Read the model definition and answer for the solid it produces. Units are mm, in the model's axes. A direction names the side the tool comes from. Coordinates: 2 decimals unless noted, no trailing zeros. Loops run counter-clockwise (first coordinate to the right, second up) from the corner with the lowest first, then second, coordinate; pieces in that order, holes last. Notation, with made-up numbers: M 6.25,0 L 23.25,0 A18 ccw 23.25,31 Z; hole C -22.5,-7.5 d8. An arc over 180 degrees is marked long. Use one line per item in the form item = value. Start each with the question number.
1. The part is cut by section B-B (x = 122.5). Give the vertices of the cut face in (y, z) (3 decimals), plus the area to 3 significant figures.
2. The part is cut by section D-D (z = -32.5). Give the vertices of the cut face in (x, y).
3. The part is cut by section A-A (y = 35). Give the vertices of the cut face in (x, z) (3 decimals), plus the area to 3 significant figures.
4. Find the intervals of material crossed by probe 1 along Z at (x, y) = (30, 36) (3 decimals); probe 2 along Y at (x, z) = (71.12, 4); probe 3 along Y at (x, z) = (71.12, 1.5), in increasing order. Write a range as [from, to].
5. For a pull along Y with two mould halves and no side action, classify faces 5 (the flat face through (35, 35, -9.525)), 6 (the cylindrical face through (166.765, 28.206, -10.671)), 7 (the flat face through (106, 31.75, -19)) as released by +Y, released by -Y, zero draft, split by the parting line, or undercut.
6. A tool of negligible diameter and unlimited length cuts with its end or side. For faces 1 (the cylindrical face through (63.684, 34.881, -27.429)), 2 (the cylindrical face through (61.597, 22.47, 4.507)), 3 (the flat face through (71.1, 6.6, 2.54)), 4 (the flat face through (84.264, 7, 4)), from which of +Z, -Z, +X, -X, +Y, -Y can it reach the whole face along a straight path? Write none if from no direction.
7. Flat-ended cylindrical pins translate along their axes: pin 1 (8 mm diameter, centred on x = 41, y = 12, fed in from +Z); pin 2 (5 mm diameter, centred on y = 34.5, z = -18.5, fed in from +X); pin 3 (10 mm diameter, centred on y = 6.5, z = 3, fed in from +X); pin 4 (5 mm diameter, centred on x = 20, z = 3.5, fed in from +Y). Find the tip coordinate at first contact, or state that the pin passes through.
from build123d import *

# Parameters (mm, degrees)
BOSS_EXTRUDE1_DEPTH = 38.1
SKETCH2_R           = 10.8585
CUT_EXTRUDE1_DEPTH  = 25.4
SKETCH3_R           = 10.8585
CUT_EXTRUDE2_DEPTH  = 25.4
FILLET1_R           = 10
FILLET2_R           = 10
SKETCH5_W           = 26.289
SKETCH5_H           = 26.289
BOSS_EXTRUDE2_DEPTH = 8.89
SKETCH6_R           = 8.0645
CUT_EXTRUDE3_DEPTH  = 6.35
SKETCH7_R           = 6.35
CUT_EXTRUDE4_DEPTH  = 5.08
FILLET3_R           = 12.7
SKETCH8_W           = 58.1046987
SKETCH8_H           = 19.05
CUT_EXTRUDE5_DEPTH  = 6.35
FILLET4_R           = 3.81


with BuildPart() as part:
    # Sketch1 → Boss-Extrude1 (new body)
    with BuildSketch(Plane(origin=(0, 0, 0), x_dir=(1, 0, 0), z_dir=(0, 1, 0))):
        Polygon((0, 0), (142.24, 0), (158.021536726, -15.781536726), (184.96230509, 11.159231637), (158.021536726, 38.1), (-15.781536726, 38.1), (-42.72230509, 11.159231637), (-15.781536726, -15.781536726), align=None)
    extrude(amount=BOSS_EXTRUDE1_DEPTH)

    # Sketch2 → Cut-Extrude1 (cut)
    with BuildSketch(Plane(origin=(-15.781536726, 0, 15.781536726), x_dir=(0.7071067811865477, 0, 0.7071067811865475), z_dir=(-0.7071067811865475, 0, 0.7071067811865477))):
        with Locations((-19.05, 19.05)):
            Circle(SKETCH2_R)
    extrude(amount=-CUT_EXTRUDE1_DEPTH, mode=Mode.SUBTRACT)

    # Sketch3 → Cut-Extrude2 (cut)
    with BuildSketch(Plane(origin=(86.901536726, 0, 86.901536726), x_dir=(0.7071067811865478, 0, -0.7071067811865474), z_dir=(0.7071067811865474, 0, 0.7071067811865478))):
        with Locations((119.628868556, 19.05)):
            Circle(SKETCH3_R)
    extrude(amount=-CUT_EXTRUDE2_DEPTH, mode=Mode.SUBTRACT)

    # Fillet1
    fillet1_edges = [part.edges().sort_by_distance(p)[0] for p in [
        (142.24, 19.05, 0),
        (0, 19.05, 0),
    ]]
    fillet(fillet1_edges, radius=FILLET1_R)

    # Fillet2
    fillet2_edges = [part.edges().sort_by_distance(p)[0] for p in [
        (-15.781536726, 19.05, -38.1),
        (158.021536726, 19.05, -38.1),
    ]]
    fillet(fillet2_edges, radius=FILLET2_R)

    # Sketch5 → Boss-Extrude2 (add)
    with BuildSketch(Plane.XY):
        with Locations((71.12, 13.1445)):
            Rectangle(SKETCH5_W, SKETCH5_H)
    extrude(amount=BOSS_EXTRUDE2_DEPTH)

    # Sketch6 → Cut-Extrude3 (cut)
    with BuildSketch(Plane.XY.offset(8.89)):
        with Locations((71.12, 13.1445)):
            Circle(SKETCH6_R)
    extrude(amount=-CUT_EXTRUDE3_DEPTH, mode=Mode.SUBTRACT)

    # Sketch7 → Cut-Extrude4 (cut)
    with BuildSketch(Plane.XY.offset(2.54)):
        with Locations((71.12, 13.1445)):
            Circle(SKETCH7_R)
    extrude(amount=-CUT_EXTRUDE4_DEPTH, mode=Mode.SUBTRACT)

    # Fillet3
    fillet3_edges = [part.edges().sort_by_distance(p)[0] for p in [
        (57.9755, 26.289, 4.445),
        (84.2645, 26.289, 4.445),
    ]]
    fillet(fillet3_edges, radius=FILLET3_R)

    # Sketch8 → Cut-Extrude5 (cut)
    with BuildSketch(Plane(origin=(0, 38.1, 0), x_dir=(1, 0, 0), z_dir=(0, 1, 0))):
        with Locations((35.71765065, 19.05)):
            Rectangle(SKETCH8_W, SKETCH8_H)
        with Locations((106.52234935, 19.05)):
            Rectangle(SKETCH8_W, SKETCH8_H)
    extrude(amount=-CUT_EXTRUDE5_DEPTH, mode=Mode.SUBTRACT)

    # Fillet4
    fillet4_edges = [part.edges().sort_by_distance(p)[0] for p in [
        (6.6653013, 34.925, -9.525),
        (6.6653013, 34.925, -28.575),
        (64.77, 34.925, -28.575),
        (64.77, 34.925, -9.525),
        (135.5746987, 34.925, -28.575),
        (135.5746987, 34.925, -9.525),
        (77.47, 34.925, -9.525),
        (77.47, 34.925, -28.575),
    ]]
    fillet(fillet4_edges, radius=FILLET4_R)


solid = part.part
Computed values:
q1.outline = M 0,-38.1 L 38.1,-38.1 L 38.1,-28.575 L 31.75,-28.575 L 31.75,-9.525 L 38.1,-9.525 L 38.1,0 L 0,0 Z
q1.area = 1,330 mm²
q2.outline = M -21.38,0 L 163.62,0 L 163.62,38.1 L -21.38,38.1 Z
q3.outline = M -42.722,-11.159 L -18.71,-35.171 A10 ccw -11.639,-38.1 L 153.879,-38.1 A10 ccw 160.95,-35.171 L 184.962,-11.159 L 158.022,15.782 L 145.169,2.929 A10 cw 138.098,0 L 4.142,0 A10 cw -2.929,2.929 L -15.782,15.782 Z; hole M 6.665,-24.765 A3.81 ccw 10.475,-28.575 L 60.96,-28.575 A3.81 ccw 64.77,-24.765 L 64.77,-13.335 A3.81 ccw 60.96,-9.525 L 10.475,-9.525 A3.81 ccw 6.665,-13.335 Z; hole M 77.47,-24.765 A3.81 ccw 81.28,-28.575 L 131.765,-28.575 A3.81 ccw 135.575,-24.765 L 135.575,-13.335 A3.81 ccw 131.765,-9.525 L 81.28,-9.525 A3.81 ccw 77.47,-13.335 Z
q3.area = 6,130 mm²
q4.probe_1 = [-38.1, -28.575], [-9.525, 0]
q4.probe_2 = [0, 5.08], [21.21, 26.29]
q4.probe_3 = [0, 6.79], [19.49, 26.29]
q5.face_5 = zero draft
q5.face_6 = undercut
q5.face_7 = released by +Y
q6.face_1 = +Y
q6.face_2 = +Z, +Y
q6.face_3 = +Z
q6.face_4 = +Z, +Y, -Y
q7.pin_1 = 0
q7.pin_2 = 180.12
q7.pin_3 = 175.8
q7.pin_4 = through
